```python
from build123d import *

# Parameters (mm, degrees)
BOSS_EXTRUDE1_DEPTH = 5


with BuildPart() as part:
    # Sketch1 → Boss-Extrude1 (new body)
    with BuildSketch(Plane(origin=(0, 0, 0), x_dir=(0, 0, -1), z_dir=(1, 0, 0))):
        Polygon((40, 50), (40, 55), (50, 55), (50, 50), (60, 50), (60, 55), (70, 55), (70, 50), (80, 50), (80, 55), (90, 55), (90, 50), (100, 50), (100, 55), (110, 55), (110, 50), (120, 50), (120, 55), (130, 55), (130, 50), (140, 50), (140, 55), (150, 55), (150, 50), (160, 50), (160, 55), (170, 55), (170, 50), (180, 50), (180, 55), (190, 55), (190, 50), (200, 50), (200, 0), (190, 0), (190, -5), (180, -5), (180, 0), (170, 0), (170, -5), (160, -5), (160, 0), (150, 0), (150, -5), (140, -5), (140, 0), (130, 0), (130, -5), (120, -5), (120, 0), (110, 0), (110, -5), (100, -5), (100, 0), (90, 0), (90, -5), (80, -5), (80, 0), (70, 0), (70, -5), (60, -5), (60, 0), (50, 0), (50, -5), (40, -5), (40, 0), (30, 0), (30, -5), (20, -5), (20, 0), (0, 0), (0, 50), (20, 50), (20, 55), (30, 55), (30, 50), align=None)
    extrude(amount=BOSS_EXTRUDE1_DEPTH)


solid = part.part
```
Geometry check sheet. Reference: the model listing, model coordinates, mm. A direction names the side the tool comes from. Coordinates: 2 decimals unless noted, no trailing zeros. Order: outer loops, then holes, each group sorted by start corner. A loop starts at its lowest first (then second) coordinate and runs counter-clockwise, first axis right, second up. Notation, with made-up numbers: (54.25, -14) - (88.25, -14) arc R15 ccw to (88.25, 15) - close; hole circle Ø3 at (66, 71). An arc over 180 degrees is marked (long way). Answer as a JSON object with one key per item and string values. Group by question number.
Item 1: Tool access check on faces 1 (the face through (2, 0, -95)), 2 (the face through (2, 53, -50)), 3 (the face through (2, 55, -125)). Record the directions out of +Z, -Z, +X, -X, +Y, -Y that give a thin tool (end or side, any length) a straight path to the whole face; none if there is none.
Item 2: Draft check along Z on faces 4 (the face through (2, 53, -190)), 5 (the face through (2, 52, -120)), 6 (the face through (2, -5, -125)). Enter one of: +Z half, -Z half, draft (parallel to the pull), parting line (faces both ways), or undercut.
Item 3: Sectioned sample at A-A, the plane z = -72.5. Record the cut outline in (x, y).
Item 4: Scan line: probe 1 along Y at (x, z) = (3.4, -110.5). Record every from-to range of solid material in increasing order.
Item 5: Depth check by flat-ended pin: pin 1 Ø2.5 at (x, y) = (1.5, 52.5) entering from -Z; pin 2 Ø1.5 at (x, y) = (3, -3) entering from +Z; pin 3 Ø2.5 at (x, z) = (2.5, -117.5) entering from +Y. Enter the tip coordinate at first touch or a pass-through.
Resolved:
{
 "1": {"face 1": "+X, -X, -Y", "face 2": "+X, -X, +Y", "face 3": "+Z, -Z, +X, -X, +Y"},
 "2": {"face 4": "-Z half", "face 5": "undercut", "face 6": "draft"},
 "3": {"outline": "(0, 0) - (5, 0) - (5, 50) - (0, 50) - close"},
 "4": {"probe 1": "0 to 50"},
 "5": {"pin 1": "z = -190", "pin 2": "z = -20", "pin 3": "y = 50"}
}
